```python
from build123d import *

# Parameters (mm, degrees)
EXTRUDE_1_DEPTH           = 6
SKETCH_6_OUTSIDE_W        = 112.61
SKETCH_6_OUTSIDE_H        = 112.61
SKETCH_6_OUTSIDE_R        = 10.5
CUT_EXTRUDE_2_DEPTH       = 10
SKETCH_7_R                = 1.2
EXTRUDE_3_DEPTH           = 5
EXTRUDE_3_DRAFT           = 1
EXTRUDE_3_PROFILE_2_DEPTH = 5
EXTRUDE_3_PROFILE_2_DRAFT = 1
EXTRUDE_3_PROFILE_3_DEPTH = 5
EXTRUDE_3_PROFILE_3_DRAFT = 1
SWEEP_1_PROFILE_R         = 0.6
PATTERN_CIRCULAR_1_COUNT  = 3


with BuildPart() as part:
    # 草图1 → 凸台-拉伸1 (new body)
    with BuildSketch(Plane(origin=(0, 0, 0), x_dir=(1, 0, 0), z_dir=(0, 1, 0))):
        with BuildLine():
            Line((-28.1, 43.1), (28.1, 43.1))
            ThreePointArc((28.1, 43.1), (38.706601718, 38.706601718), (43.1, 28.1))
            Line((43.1, 28.1), (43.1, -28.1))
            ThreePointArc((43.1, -28.1), (38.706601718, -38.706601718), (28.1, -43.1))
            Line((28.1, -43.1), (-28.1, -43.1))
            ThreePointArc((-28.1, -43.1), (-38.706601718, -38.706601718), (-43.1, -28.1))
            Line((-43.1, -28.1), (-43.1, 28.1))
            ThreePointArc((-43.1, 28.1), (-38.706601718, 38.706601718), (-28.1, 43.1))
        make_face()
    extrude(amount=EXTRUDE_1_DEPTH)

    # 草图6 outside → 切除-拉伸2 (cut)
    with BuildSketch(Plane(origin=(0, 6, 0), x_dir=(1, 0, 0), z_dir=(0, 1, 0))):
        Rectangle(SKETCH_6_OUTSIDE_W, SKETCH_6_OUTSIDE_H)
        with Locations(Location((0, 0, 0), (0, 0, 270))):
            Circle(SKETCH_6_OUTSIDE_R, mode=Mode.SUBTRACT)
    extrude(amount=-CUT_EXTRUDE_2_DEPTH, mode=Mode.SUBTRACT)


with BuildPart() as extrude_3_tool:
    # 草图7 → 凸台-拉伸3 (with draft: the straight prism first)
    with BuildSketch(Plane.XZ):
        with Locations((8.5, 0)):
            Circle(SKETCH_7_R)
    extrude(amount=EXTRUDE_3_DEPTH)
    # 凸台-拉伸3: the draft: its side faces are tilted about the plane it starts from
    extrude_3_sides = [extrude_3_tool.faces().sort_by_distance(p)[0] for p in [
        (7.3, -2.5, 0),
    ]]
    draft(extrude_3_sides, Plane.XZ, EXTRUDE_3_DRAFT)


with BuildPart() as part_1:
    add(part.part)

    # 凸台-拉伸3: add extrude_3_tool
    add(extrude_3_tool.part)


with BuildPart() as extrude_3_profile_2_tool:
    # 草图7 → 凸台-拉伸3 profile 2 (with draft: the straight prism first)
    with BuildSketch(Plane.XZ):
        with Locations((-4.25, -7.361215932)):
            Circle(SKETCH_7_R)
    extrude(amount=EXTRUDE_3_PROFILE_2_DEPTH)
    # 凸台-拉伸3 profile 2: the draft: its side faces are tilted about the plane it starts from
    extrude_3_profile_2_sides = [extrude_3_profile_2_tool.faces().sort_by_distance(p)[0] for p in [
        (-5.45, -2.5, -7.361215932),
    ]]
    draft(extrude_3_profile_2_sides, Plane.XZ, EXTRUDE_3_PROFILE_2_DRAFT)


with BuildPart() as part_2:
    add(part_1.part)

    # 凸台-拉伸3 profile 2: add extrude_3_profile_2_tool
    add(extrude_3_profile_2_tool.part)


with BuildPart() as extrude_3_profile_3_tool:
    # 草图7 → 凸台-拉伸3 profile 3 (with draft: the straight prism first)
    with BuildSketch(Plane.XZ):
        with Locations((-4.25, 7.361215932)):
            Circle(SKETCH_7_R)
    extrude(amount=EXTRUDE_3_PROFILE_3_DEPTH)
    # 凸台-拉伸3 profile 3: the draft: its side faces are tilted about the plane it starts from
    extrude_3_profile_3_sides = [extrude_3_profile_3_tool.faces().sort_by_distance(p)[0] for p in [
        (-5.45, -2.5, 7.361215932),
    ]]
    draft(extrude_3_profile_3_sides, Plane.XZ, EXTRUDE_3_PROFILE_3_DRAFT)


with BuildPart() as part_3:
    add(part_2.part)

    # 凸台-拉伸3 profile 3: add extrude_3_profile_3_tool
    add(extrude_3_profile_3_tool.part)

    # 草图8 → 切除-旋转1 (revolve, cut)
    with BuildSketch(Plane(origin=(0, 9.5, 0), x_dir=(1, 0, 0), z_dir=(0, 1, 0))):
        with BuildLine():
            Line((0, 6), (0, -6))
            ThreePointArc((0, -6), (-6, 0), (0, 6))
        make_face()
    revolve(axis=Axis((0, 9.5, -6), (0, 0, 1)), mode=Mode.SUBTRACT)

    # 切除-拉伸3 cone 1 section (through the dimple's axis) → 切除-拉伸3 (revolve, cut)
    with BuildSketch(Plane(origin=(0, 0, 0), x_dir=(0, 0, -1), z_dir=(1, 0, 0))):
        Polygon((0, 0), (6, 0), (0, 2.06596568), align=None)
    revolve(axis=Axis((0, 0, 0), (0, 1, 0)), mode=Mode.SUBTRACT)

    # 切除-扫描1: sweep along a path in 草图12
    with BuildLine(Plane(origin=(0, 0, 0), x_dir=(0, 0, -1), z_dir=(1, 0, 0))) as sweep_1_path:
        Line((-3.177240677, 6.426747641), (-5.652840705, -1.383969025))
    # 切除-扫描1 profile (on start of the path) → 切除-扫描1 (sweep, cut)
    with BuildSketch(Plane(origin=(0, 6.426747641, 3.177240677), x_dir=(0, -0.30213643640779364, -0.9532646924096158), z_dir=(0, -0.9532646924096158, 0.30213643640779364))):
        Circle(SWEEP_1_PROFILE_R)
    sweep_1 = sweep(path=sweep_1_path.line, mode=Mode.SUBTRACT)

    # 阵列(圆周)1: 切除-扫描1 ×3 about axis
    pattern_circular_1_axis = Axis((0, 6, 0), (0, 1, 0))
    for i in range(1, PATTERN_CIRCULAR_1_COUNT):
        add(sweep_1.rotate(pattern_circular_1_axis, i * 360 / PATTERN_CIRCULAR_1_COUNT), mode=Mode.SUBTRACT)


solid = part_3.part
```
Input: part model. Units: mm. Frame: model coordinates. A direction names the side the tool comes from. Give positions to 0.01 mm unless a question says otherwise; leave off trailing zeros. Loops run counter-clockwise (first coordinate to the right, second up) from the corner with the lowest first, then second, coordinate; pieces in that order, holes last. Notation, with made-up numbers: (61.5, 57) -> (120.5, 57) arc R32 cw to (120.5, 86) -> close; hole circle Ø9 at (-34.5, 40). An arc over 180 degrees is marked (long way). Use a Markdown table: item, result.
Q1. Pull-direction query (X, two-part tool) for faces 3 (the cylindrical face through (3.2, 3, 10)), 4 (the flat face through (8, -5, 0)), 5 (the conical face through (0.177, 1.966, 0.231)); classes: pulls with the +X half, pulls with the -X half, needs draft (parallel to the pull), parting line crosses it, or undercut.
Entries:
| item | result |
|---|---|
| face 3 | parting line crosses it |
| face 4 | needs draft |
| face 5 | undercut |
Q2. Section query A-A, the plane y = -3.75. Return the cut outline in (x, z), plus the area to 3 significant figures.
Entries:
| item | result |
|---|---|
| outline | circle Ø2.27 at (-4.25, -7.36); circle Ø2.27 at (-4.25, 7.36); circle Ø2.27 at (8.5, 0) |
| area | 12.1 mm² |
Q3. Ray query, probe 1 along Y at (x, z) = (0.75, 7.25); probe 2 along Z at (x, y) = (3.5, 2.5); probe 3 along X at (y, z) = (5.5, 8.5). Return the intervals inside material, ascending. Write a range as from..to.
Entries:
| item | result |
|---|---|
| probe 1 | y = 0..6 |
| probe 2 | z = -9.9..-2.71, -1.68..9.9 |
| probe 3 | x = -6.16..6.16 |
Q4. Access query for faces 1 (the conical face through (-5.406, -2.465, -7.31)), 2 (the cylindrical face through (0.03, 2.6, 5.02)). Directions: +Z, -Z, +X, -X, +Y, -Y. A direction counts if a zero-diameter tool reaches every point of the face in a straight line with its end or side. Return the directions, or none.
Entries:
| item | result |
|---|---|
| face 1 | -Y |
| face 2 | none |
Q5. First-contact query: P1, Ø1, axis at y = 4, z = 8, coming from the -X side; P2, Ø8, axis at x = -3.5, z = 0, coming from the -Y side; P3, Ø2, axis at x = -7, y = 0.5, coming from the -Z side. Flat tips, straight axial feed; report the tip coordinate or a pass-through.
Entries:
| item | result |
|---|---|
| P1 | stops at x = -7.35 |
| P2 | stops at y = 0 |
| P3 | stops at z = -8.62 |
